The drawing under review shows one solid part. Ordinate dimensions are in mm from its lowest x, y, z. A direction names the side the tool comes from. Coordinates: 2 decimals unless noted, no trailing zeros. Loops run counter-clockwise (first coordinate to the right, second up) from the corner with the lowest first, then second, coordinate; pieces in that order, holes last. Notation, with made-up numbers: (22.5, 41) -> (56.5, 41) arc R13 cw to (56.5, 46) -> close; hole circle Ø9 at (43, -10.75). An arc over 180 degrees is marked (long way). Use a Markdown table: item, result.
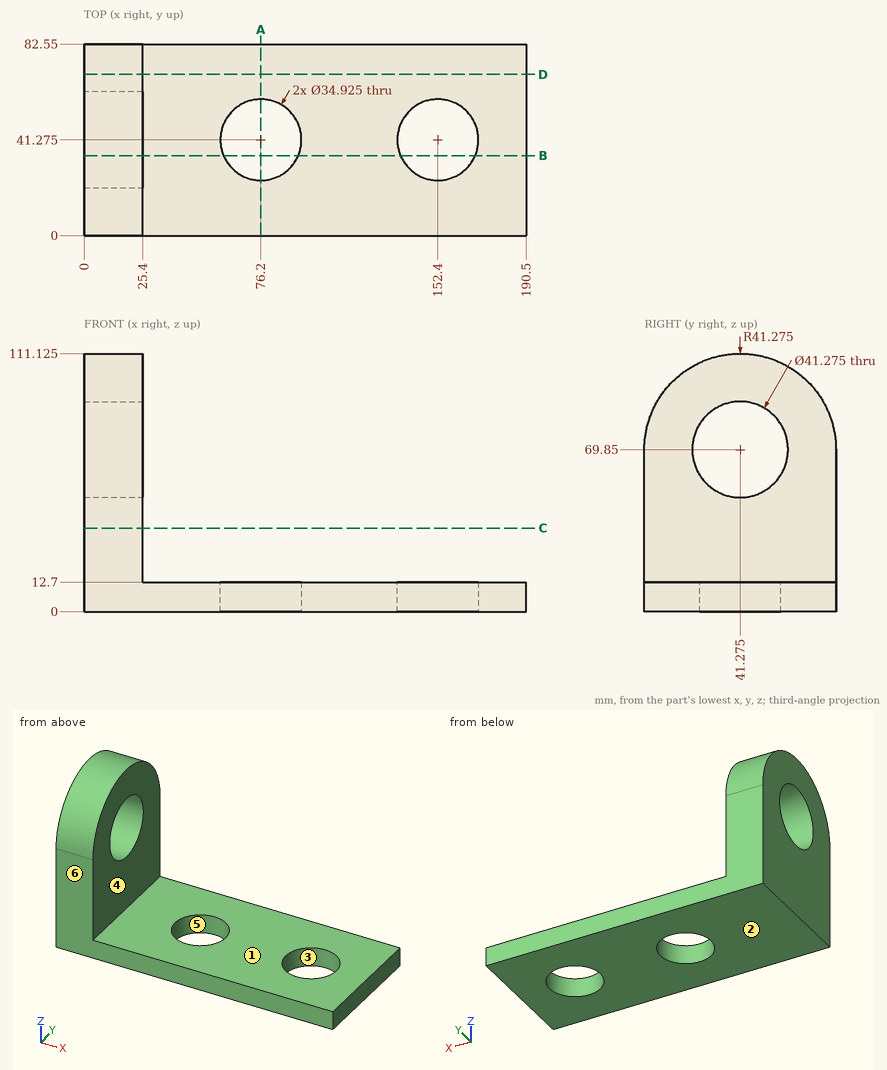
(1) Mouldability with a two-part tool opening along X and no side actions: class the marked faces 3, 4, 5 and 6 as pulls with the +X half, pulls with the -X half, needs draft (parallel to the pull), parting line crosses it, or undercut.
Found:
| item | result |
|---|---|
| face 3 | undercut |
| face 4 | pulls with the +X half |
| face 5 | undercut |
| face 6 | needs draft |
(2) For pin 1 Ø5 at (y, z) = (25.5, 31) entering from +X; pin 2 Ø25 at (y, z) = (41.275, 69.85) entering from -X, all flat-tipped, find the tip position at first contact; note any pin that passes through.
Found:
| item | result |
|---|---|
| pin 1 | stops at x = 25.4 |
| pin 2 | passes through |
(3) Take a section at A-A on x = 76.2. Write out the cut boundary in (y, z), plus the area to 3 significant figures.
Found:
| item | result |
|---|---|
| outline | (0, 0) -> (23.81, 0) -> (23.81, 12.7) -> (0, 12.7) -> close; (58.74, 0) -> (82.55, 0) -> (82.55, 12.7) -> (58.74, 12.7) -> close |
| area | 605 mm^2 |
(4) For the marked faces 1 and 2, list the 3-axis set-ups (+Z, -Z, +X, -X, +Y, -Y) from which the entire face can be reached by the end or side of a thin tool; tool diameter is ignored.
Found:
| item | result |
|---|---|
| face 1 | +Z, +X, +Y, -Y |
| face 2 | -Z, +X, -X, +Y, -Y |
(5) Take a section at B-B on y = 34.5. Write out the cut boundary in (x, z), plus the area to 3 significant figures.
Found:
| item | result |
|---|---|
| outline | (0, 0) -> (60.11, 0) -> (60.11, 12.7) -> (25.4, 12.7) -> (25.4, 50.36) -> (0, 50.36) -> close; (0, 89.34) -> (25.4, 89.34) -> (25.4, 110.57) -> (0, 110.57) -> close; (92.29, 0) -> (136.31, 0) -> (136.31, 12.7) -> (92.29, 12.7) -> close; (168.49, 0) -> (190.5, 0) -> (190.5, 12.7) -> (168.49, 12.7) -> close |
| area | 3,100 mm^2 |
(6) For line 1 along Y through (x, z) = (76.2, 6.5); line 2 along Y through (x, z) = (8, 69); line 3 along Z through (x, y) = (47, 36), list the stretches that pass through material, from the lowest coordinate up.
Found:
| item | result |
|---|---|
| line 1 | y = 0 to 23.81, 58.74 to 82.55 |
| line 2 | y = 0 to 20.66, 61.89 to 82.55 |
| line 3 | z = 0 to 12.7 |
(7) Take a section at D-D on y = 69.5. Write out the cut boundary in (x, z), plus the area to 3 significant figures.
Found:
| item | result |
|---|---|
| outline | (0, 0) -> (190.5, 0) -> (190.5, 12.7) -> (25.4, 12.7) -> (25.4, 99.97) -> (0, 99.97) -> close |
| area | 4,640 mm^2 |
(8) Take a section at C-C on z = 36. Write out the cut boundary in (x, y).
Found:
| item | result |
|---|---|
| outline | (0, 0) -> (25.4, 0) -> (25.4, 82.55) -> (0, 82.55) -> close |
